Autodesk Inventor part; units mm, degrees
ref_plane "YZ Plane" through (0, 0, 0) normal (1, 0, 0) x (0, 1, 0)
ref_plane "XZ Plane" through (0, 0, 0) normal (0, 1, 0) x (-1, 0, 0)
ref_plane "XY Plane" through (0, 0, 0) normal (0, 0, 1) x (1, 0, 0)
sketch "Эскиз1" plane through (0, 0, 0) normal (0, 0, 1) x (1, 0, 0)
  circle A0 centre (0, 0) radius 22.47
  line L0 (21.9066, 5) -> (21.9066, -5)
  circle A1 centre (21.9066, -5) radius 2.05
  circle A2 centre (21.9066, 5) radius 2.05
  line L1 (21.9066, 5) -> (0, 0)
  line L2 (0, 0) -> (21.9066, -5)
  line L3 (21.9066, 5) -> (13.9325, -4.5032)
  circle A3 centre (0, 0) radius 15.4921
  line L4 (20.5889, 3.4296) -> (24.3782, 0.25)
  line L5 (0, 0) -> (4.0279, 0)
  line L6 (20.5889, -3.4296) -> (24.3782, -0.25)
  line L7 (24.3782, 0.25) -> (24.3782, -0.25)
  line L8 (21.9066, -5) -> (14.1251, 4.2737)
  line L9 (21.8556, 10.8026) -> (22.0725, 10.3521)
  circle A4 centre (21.9066, 5.0001) radius 2.05
  line L10 (20.038, 5.8432) -> (22.0725, 10.3521)
  line L11 (17.0619, 12.0232) -> (21.8556, 10.8026)
  circle A5 centre (17.5678, 14.0098) radius 2.05
  line L12 (15.0041, 19.2155) -> (15.395, 18.9038)
  circle A6 centre (17.5677, 14.0099) radius 2.05
  line L13 (15.5184, 13.9587) -> (15.395, 18.9038)
  line L14 (10.1556, 18.2354) -> (15.0041, 19.2155)
  circle A7 centre (9.7494, 20.2448) radius 2.05
  line L15 (5.1809, 23.8227) -> (5.6684, 23.7114)
  circle A8 centre (9.7493, 20.2448) radius 2.05
  line L16 (7.9251, 19.3096) -> (5.6684, 23.7114)
  line L17 (1.2378, 20.8359) -> (5.1809, 23.8227)
  circle A9 centre (0, 22.47) radius 2.05
  line L18 (-5.6684, 23.7114) -> (-5.1809, 23.8227)
  circle A10 centre (0, 22.47) radius 2.05
  line L19 (-1.2378, 20.8359) -> (-5.1809, 23.8227)
  line L20 (-7.9251, 19.3096) -> (-5.6684, 23.7114)
  circle A11 centre (-9.7493, 20.2448) radius 2.05
  line L21 (-15.395, 18.9038) -> (-15.0041, 19.2155)
  circle A12 centre (-9.7494, 20.2448) radius 2.05
  line L22 (-10.1556, 18.2354) -> (-15.0041, 19.2155)
  line L23 (-15.5184, 13.9587) -> (-15.395, 18.9038)
  circle A13 centre (-17.5677, 14.0099) radius 2.05
  line L24 (-22.0725, 10.3521) -> (-21.8556, 10.8026)
  circle A14 centre (-17.5678, 14.0098) radius 2.05
  line L25 (-17.0619, 12.0232) -> (-21.8556, 10.8026)
  line L26 (-20.038, 5.8432) -> (-22.0725, 10.3521)
  circle A15 centre (-21.9066, 5.0001) radius 2.05
  line L27 (-24.3782, -0.25) -> (-24.3782, 0.25)
  circle A16 centre (-21.9066, 5) radius 2.05
  line L28 (-20.5889, 3.4296) -> (-24.3782, 0.25)
  line L29 (-20.5889, -3.4296) -> (-24.3782, -0.25)
  circle A17 centre (-21.9066, -5) radius 2.05
  line L30 (-21.8556, -10.8026) -> (-22.0725, -10.3521)
  circle A18 centre (-21.9066, -5.0001) radius 2.05
  line L31 (-20.038, -5.8432) -> (-22.0725, -10.3521)
  line L32 (-17.0619, -12.0232) -> (-21.8556, -10.8026)
  circle A19 centre (-17.5678, -14.0098) radius 2.05
  line L33 (-15.0041, -19.2155) -> (-15.395, -18.9038)
  circle A20 centre (-17.5677, -14.0099) radius 2.05
  line L34 (-15.5184, -13.9587) -> (-15.395, -18.9038)
  line L35 (-10.1556, -18.2354) -> (-15.0041, -19.2155)
  circle A21 centre (-9.7494, -20.2448) radius 2.05
  line L36 (-5.1809, -23.8227) -> (-5.6684, -23.7114)
  circle A22 centre (-9.7493, -20.2448) radius 2.05
  line L37 (-7.9251, -19.3096) -> (-5.6684, -23.7114)
  line L38 (-1.2378, -20.8359) -> (-5.1809, -23.8227)
  circle A23 centre (0, -22.47) radius 2.05
  line L39 (5.6684, -23.7114) -> (5.1809, -23.8227)
  circle A24 centre (0, -22.47) radius 2.05
  line L40 (1.2378, -20.8359) -> (5.1809, -23.8227)
  line L41 (7.9251, -19.3096) -> (5.6684, -23.7114)
  circle A25 centre (9.7493, -20.2448) radius 2.05
  line L42 (15.395, -18.9038) -> (15.0041, -19.2155)
  circle A26 centre (9.7494, -20.2448) radius 2.05
  line L43 (10.1556, -18.2354) -> (15.0041, -19.2155)
  line L44 (15.5184, -13.9587) -> (15.395, -18.9038)
  circle A27 centre (17.5677, -14.0099) radius 2.05
  line L45 (22.0725, -10.3521) -> (21.8556, -10.8026)
  circle A28 centre (17.5678, -14.0098) radius 2.05
  line L46 (17.0619, -12.0232) -> (21.8556, -10.8026)
  line L47 (20.038, -5.8432) -> (22.0725, -10.3521)
  circle A29 centre (21.9066, -5.0001) radius 2.05
  line L48 (22.3878, 1.9202) -> (22.3878, -1.9202)
  circle A30 centre (0, 0) radius 11.3
  point P0 (21.9066, 0)
  point P1 (19.908, 4.5439)
  point P2 (15.965, 12.7317)
  point P3 (8.8599, 18.3978)
  point P4 (0, 20.42)
  point P5 (-8.8599, 18.3978)
  point P6 (-15.965, 12.7317)
  point P7 (-19.908, 4.5439)
  point P8 (-19.908, -4.5439)
  point P9 (-15.965, -12.7317)
  point P10 (-8.8599, -18.3978)
  point P11 (0, -20.42)
  point P12 (8.8599, -18.3978)
  point P13 (15.965, -12.7317)
  point P14 (19.908, -4.5439)
  point P15 (11.0167, -2.5145)
  point P16 (11.0167, 2.5145)
  point P17 (15.1037, 3.4473)
  point P18 (15.1037, -3.4473)
  dimension "d3" = 4.1
  dimension "d0" = 44.94
  dimension "d1" = 10
  dimension "d2" = 4.1
  dimension "d4" = 40
  dimension "d6" = 40
  dimension "d9" = 360
  dimension "d13" = 0.5
  dimension "d23" = 3.8403
  dimension "d24" = 22.6
extrude "Выдавливание1" add sketch "Эскиз1" along normal blind 3.7 contours A0 L48 | A0 L4 L7 L6 | L48 L6 L0 L4 | L0 L6 L8 L3 L4 | L3 L8 A3 L1 A2 | A1 L2 A3 L3 L8 | L1 A3 L2 A1 L47 A0 L46 A27 L44 L43 A25 L41 L40 A23 L38 L37 A21 L35 L34 A19 L32 L31 A17 L29 L28 A15 L26 L25 A13 L23 L22 A11 L20 L19 A9 L17 L16 A7 L14 L13 A5 L11 L10 A2 | L3 A3 L8 | A0 L11 L9 L10 | A3 L8 L1 | L1 A30 L2 A3 | A3 L2 L3 | L3 L2 A30 L1 L8 A3 | L47 L45 L46 A0 | A0 L14 L12 L13 | L44 L42 L43 A0 | A0 L17 L15 L16 | L41 L39 L40 A0 | A0 L20 L18 L19 | L38 L36 L37 A0 | A0 L23 L21 L22 | L35 L33 L34 A0 | A0 L26 L24 L25 | L32 L30 L31 A0 | A0 L29 L27 L28
sketch "Эскиз5" plane through (0, 0, 3.7) normal (0, 0, 1) x (1, 0, 0)
  circle A0 centre (0, 0) radius 13.8
  circle A1 centre (0, 0) radius 11.3
  dimension "d25" = 2.5
extrude "Выдавливание3" add sketch "Эскиз5" along normal blind 22.4
sketch "Эскиз6" plane through (0, 0, 26.1) normal (0, 0, 1) x (1, 0, 0)
  circle A0 centre (0, 0) radius 13.8
  circle A1 centre (-1.995, 7.7473) radius 1.55
  circle A2 centre (7.7068, -2.1459) radius 1.55
  circle A3 centre (-5.7118, -5.6014) radius 1.55
extrude "Выдавливание4" add sketch "Эскиз6" along normal blind 3
sketch "Эскиз7" plane through (0, 0, 29.1) normal (0, 0, 1) x (1, 0, 0)
  circle A0 centre (0, 0) radius 11.3
  circle A1 centre (0, 0) radius 13.8
extrude "Выдавливание5" add sketch "Эскиз7" along normal blind 17.3
equation "\"d2\" = d3"
properties part number "ВедущееКолесо" material "Пластик ЖКП"
Check sheet for the modelled part. Datum: model origin and axes. Units: mm. A direction names the side the tool comes from. Coordinates: 2 decimals unless noted, no trailing zeros. Write each loop counter-clockwise with the first axis right and the second up, starting at its lowest first coordinate (ties: lowest second). Pieces come first, ordered by that corner, then holes. Notation, with made-up numbers: M 67.25,11 L 125.25,11 A19 ccw 125.25,27 Z; hole C 41.25,1 d9. An arc over 180 degrees is marked long. Write item = value, one per line. Start each with the question number.
1. Sectioned sample at D-D (y = 15). Record the cut outline in (x, z).
2. Mould release check, pull along X, two halves, no side actions. Record for faces 1 (the flat face through (-6.8, 21.5, 1.8)), 2 (the cylindrical face through (15.95, -12.75, 1.82)), 3 (the cylindrical face through (-6.05, -4.09, 27.58)): pulls with the +X half, pulls with the -X half, needs draft (parallel to the pull), parting line crosses it, or undercut.
3. Sectioned sample at C-C (z = 20.5). Record the cut outline in (x, y).
4. Thickness scan on probe 1 along X at (y, z) = (0.5, 13); probe 2 along Y at (x, z) = (0, 35); probe 3 along Z at (x, y) = (-4.5, -16.5). Record the ranges inside material, lowest first.
5. Sectioned sample at A-A (x = -9). Record the cut outline in (y, z), then the cut area to 3 significant figures.
6. Tool access check on faces 4 (the cylindrical face through (10.78, -3.39, 12.87)), 5 (the flat face through (22.46, -1.86, 1.82)), 6 (the cylindrical face through (-1.796, -13.683, 24.751)). Record the directions out of +Z, -Z, +X, -X, +Y, -Y that give a thin tool (end or side, any length) a straight path to the whole face; none if there is none.
7. Sectioned sample at B-B (y = 2). Record the cut outline in (x, z).
8. Go/stop test with flat-tipped pins: pin 1 (10 mm diameter, centred on x = 9.5, z = 36.5, fed in from -Y); pin 2 (3.5 mm diameter, centred on x = -2, y = 7.75, fed in from +Z); pin 3 (3 mm diameter, centred on y = 12.5, z = 26, fed in from +X); pin 4 (6 mm diameter, centred on x = -18, z = 34.5, fed in from -Y). Record where each tip stops, or that it passes through.
The answers:
q1.outline = M -15.49,0 L 15.49,0 L 15.49,3.7 L -15.49,3.7 Z
q2.face_1 = pulls with the -X half
q2.face_2 = pulls with the +X half
q2.face_3 = undercut
q3.outline = C 0,0 d27.6; hole C 0,0 d22.6
q4.probe_1 = -13.79 to -11.29, 11.29 to 13.79
q4.probe_2 = -13.8 to -11.3, 11.3 to 13.8
q4.probe_3 = 0 to 3.7
q5.outline = M -18.34,0 L -6.83,0 L -6.83,26.1 L 6.83,26.1 L 6.83,0 L 18.34,0 L 18.34,3.7 L 10.46,3.7 L 10.46,46.4 L 6.83,46.4 L 6.83,29.1 L -6.83,29.1 L -6.83,46.4 L -10.46,46.4 L -10.46,3.7 L -18.34,3.7 Z
q5.area = 436 mm²
q6.face_4 = -Z
q6.face_5 = +Z, -Z, +X
q6.face_6 = +Z
q7.outline = M -22.29,0 L -11.12,0 L -11.12,26.1 L 11.12,26.1 L 11.12,0 L 22.29,0 L 22.29,3.7 L 13.65,3.7 L 13.65,46.4 L 11.12,46.4 L 11.12,29.1 L -11.12,29.1 L -11.12,46.4 L -13.65,46.4 L -13.65,3.7 L -22.29,3.7 Z
q8.pin_1 = -13.05
q8.pin_2 = 29.1
q8.pin_3 = 8.33
q8.pin_4 = through
